Geometry: final body of the model. Coordinates: model frame, mm. Face numbers are marked on the shaded views. A direction names the side the tool comes from. Round coordinates to 2 decimals unless told otherwise and drop trailing zeros. Order: outer loops, then holes, each group sorted by start corner. A loop starts at its lowest first (then second) coordinate and runs counter-clockwise, first axis right, second up. Notation, with made-up numbers: (23, 33.5) - (81, 33.5) arc R17 ccw to (81, 44.5) - close; hole circle Ø5 at (49.25, 59.5). An arc over 180 degrees is marked (long way). Put each result on its own line as item: value. Start each with the question number.
(1) Section B-B (x = 66). Output: boundary loops of the cut face in (y, z).
(2) Section A-A (x = 89). Output: boundary loops of the cut face in (y, z), and give its area (3 significant figures).
(3) Access query for the marked faces 3 and 4. Directions: +Z, -Z, +X, -X, +Y, -Y. A direction counts if a zero-diameter tool reaches every point of the face in a straight line with its end or side. Return the directions, or none.
(4) Material intervals for L1, parallel to Z at x = 110.35, y = 0; L2, parallel to Y at x = 28.5, z = 0, sorted ascending. Write a range as [from, to].
(5) Pull-direction query (Z, two-part tool) for the marked faces 1 and 2; classes: released by +Z, released by -Z, zero draft, split by the parting line, or undercut.
(6) Pin query (flat end, axial travel): P1, Ø15, axis at y = 0, z = 0, coming from the +X side; P2, Ø10, axis at y = 25, z = 0, coming from the -X side; P3, Ø8, axis at x = 65, z = -5, coming from the -Y side; P4, Ø1.5, axis at x = 70.5, y = 7.5, coming from the -Z side. Return the tip coordinate at first contact, or that it passes through.
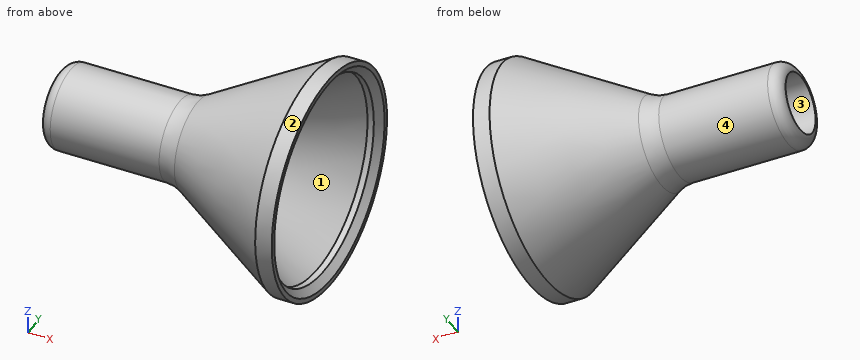
from build123d import *

# Parameters (mm, degrees)
F2_SIZE = 3
F3_R    = 15
F4_R    = 4.99999


# Not quite as in the source:
# - a fillet or chamfer is up to 0.001 mm smaller than in the source, because OpenCascade refuses the exact size


with BuildPart() as f1:
    # F0 (on Front) → F1 (revolve)
    with BuildSketch(Plane.XZ):
        Polygon((55, 17.3), (0, 17.3), (0, 12.3), (56.3397459622, 12.3), (108.3012701892, 42.3), (113.9615242271, 42.3), (113.9615242271, 47.3), (106.9615242271, 47.3), align=None)
    revolve(axis=Axis((19.2044641059, 0, 0), (1, 0, 0)))

    # F2
    f2_edges = [f1.edges().sort_by_distance(p)[0] for p in [
        (113.961524, 0, -42.3),
    ]]
    chamfer(f2_edges, length=F2_SIZE)

    # F3
    f3_edges = [f1.edges().sort_by_distance(p)[0] for p in [
        (55, 0, -17.3),
    ]]
    fillet(f3_edges, radius=F3_R)

    # F4 (radius 5 in the source; OpenCascade refuses exactly that, so slightly less here)
    f4_edges = [f1.edges().sort_by_distance(p)[0] for p in [
        (0, 0, -17.3),
    ]]
    fillet(f4_edges, radius=F4_R)


solid = f1.part
Checks:
1. outline: circle Ø47.3 at (0, 0); hole circle Ø35.75 at (0, 0)
2. outline: circle Ø73.86 at (0, 0); hole circle Ø62.31 at (0, 0)
2. area: 1,230 mm²
3. face 3: +X, -X
3. face 4: -X
4. L1: z = [-47.3, -42.3], [42.3, 47.3]
4. L2: y = [-17.3, -12.3], [12.3, 17.3]
5. face 1: undercut
5. face 2: split by the parting line
6. P1: passes through
6. P2: stops at x = 59.68
6. P3: stops at y = -24.99
6. P4: stops at z = -25.65
